Autodesk Fusion 360 part; units mm, degrees
sketch "Sketch6" plane through (0, 0, 0) normal (0, 1, 0) x (1, 0, 0)
  line L0 (0, 0) -> (-31.75, 0)
  line L1 (-31.75, 0) -> (-31.75, -7.62)
  line L2 (-31.75, -7.62) -> (0, -7.62)
  line L3 (0, -7.62) -> (0, 0)
  dimension "d16" = 7.62
  dimension "d17" = 31.75
extrude "Extrude5" add sketch "Sketch6" along normal blind 3
sketch "Sketch7" plane through (0, 0, 0) normal (0, -1, 0) x (1, 0, 0)
  line L0 (0, 0) -> (0, 7.62)
  line L1 (0, 7.62) -> (-31.75, 7.62)
  line L2 (-31.75, 7.62) -> (-31.75, 0)
  line L3 (-31.75, 0) -> (0, 0)
  circle A0 centre (-29.21, 4) radius 1.5
  circle A1 centre (-2.54, 3.81) radius 1.5
  line L4 (-31.75, 7.62) -> (-26.75, 7.62)
  line L5 (-26.75, 7.62) -> (-26.75, 0)
  line L6 (-26.75, 0) -> (-31.75, 0)
  line L7 (-31.75, 0) -> (-31.75, 7.62)
  line L8 (0, 0) -> (-5, 0)
  line L9 (-5, 0) -> (-5, 7.62)
  line L10 (-5, 7.62) -> (0, 7.62)
  line L11 (0, 7.62) -> (0, 0)
  line L12 (-31.75, 7.62) -> (-21.75, 7.62)
  line L13 (-21.75, 7.62) -> (-21.75, 0)
  line L14 (-21.75, 0) -> (-31.75, 0)
  line L15 (-31.75, 0) -> (-31.75, 7.62)
  line L16 (0, 0) -> (-10, 0)
  line L17 (-10, 0) -> (-10, 7.62)
  line L18 (-10, 7.62) -> (0, 7.62)
  line L19 (0, 7.62) -> (0, 0)
  dimension "d20" = 3
  dimension "d21" = 3
  dimension "d22" = 26.67
  dimension "d24" = 2.54
  dimension "d25" = 3.81
  dimension "d30" = 5
  dimension "d31" = 5
  dimension "d36" = 10
  dimension "d37" = 10
extrude "Extrude8" cut sketch "Sketch7" against normal blind 1 contours L1 L2 L3 L4 L5 L6 L7 L12 L14 L15
extrude "Extrude7" cut sketch "Sketch7" against normal blind 3 contours A1
extrude "Extrude6" cut sketch "Sketch7" against normal blind 3 contours A0
extrude "Extrude9" cut sketch "Sketch7" against normal blind 1 contours L0 L1 L3 L8 L9 L10 L11 L16 L18 L19
sketch "Sketch8" plane through (0, 3, 0) normal (0, 1, 0) x (-1, 0, 0)
  circle A0 centre (29.21, 4) radius 1.5
  circle A1 centre (2.54, 3.81) radius 1.5
  line L0 (0, 7.62) -> (0, 0)
  line L1 (0, 0) -> (31.75, 0)
  line L2 (31.75, 0) -> (31.75, 7.62)
  line L3 (31.75, 7.62) -> (0, 7.62)
sketch "Sketch9" plane through (0, 0, 7.62) normal (0, 0, 1) x (-1, 0, 0)
  line L0 (5, -1) -> (0, -1)
  line L1 (0, -1) -> (0, -3)
  line L2 (0, -3) -> (31.75, -3)
  line L3 (31.75, -3) -> (31.75, -1)
  line L4 (31.75, -1) -> (26.75, -1)
  line L5 (26.75, -1) -> (26.75, 0)
  line L6 (26.75, 0) -> (5, 0)
  line L7 (5, 0) -> (5, -1)
  line L8 (31.75, -3) -> (21.75, -3)
  line L9 (21.75, -3) -> (21.75, -2)
  line L10 (21.75, -2) -> (31.75, -2)
  line L11 (31.75, -2) -> (31.75, -3)
  line L12 (0, -3) -> (10, -3)
  line L13 (10, -3) -> (10, -2)
  line L14 (10, -2) -> (0, -2)
  line L15 (0, -2) -> (0, -3)
  line L16 (21.75, -3) -> (10, -3)
  line L17 (10, -3) -> (10, -2)
  line L18 (10, -2) -> (21.75, -2)
  line L19 (21.75, -2) -> (21.75, -3)
  line L20 (21.75, 0) -> (10, 0)
  line L21 (10, 0) -> (10, -1)
  line L22 (10, -1) -> (21.75, -1)
  line L23 (21.75, -1) -> (21.75, 0)
  dimension "d39" = 10
  dimension "d40" = 1
  dimension "d45" = 11.75
extrude "Extrude12" add sketch "Sketch9" along normal blind 9 contours L6 L20 L21 L22 L23
extrude "Extrude11" cut sketch "Sketch9" against normal blind 10 contours L1 L2 L12 L13 L14 L15 L17
extrude "Extrude10" cut sketch "Sketch9" against normal blind 10 contours L2 L3 L8 L9 L10 L11 L19
The listing builds one solid part. Answer for the finished solid, in the listing's coordinates (mm). A direction names the side the tool comes from. Coordinates: 2 decimals unless noted, no trailing zeros. Order: outer loops, then holes, each group sorted by start corner. A loop starts at its lowest first (then second) coordinate and runs counter-clockwise, first axis right, second up. Notation, with made-up numbers: (64.25, 14) -> (96.25, 14) arc R20 ccw to (96.25, 40) -> close; hole circle Ø7 at (-9.75, -25.5). An arc over 180 degrees is marked (long way). Answer in a Markdown table with one row per item. Add a question column.
Item 1: Each of these flat-tipped pins is pushed along its axis until it touches: P1, Ø2.5, axis at x = -30.5, z = 3.5, coming from the -Y side; P2, Ø1.5, axis at x = -15.5, z = 12, coming from the +Y side; P3, Ø4, axis at x = -2.54, z = 3.81, coming from the +Y side. Where does it stop, or does it pass through?
Item 2: Find section A-A (y = 0.4). Write down the section's boundary in (x, z), then the cut area to 3 significant figures.
Item 3: Find section B-B (x = -29.21). Write down the section's boundary in (y, z).
Item 4: Which of the six approach directions +Z, -Z, +X, -X, +Y, -Y give full straight-line access (tool end or side, diameter ignored) to faces 1 (the face through (-26.75, 0.5, 3.9)), 2 (the face through (-27, 2, 4)), 3 (the face through (-21.75, 0.5, 12.1)), 4 (the face through (-16, 1, 12)), 5 (the face through (-4.2, 1, 3.9))?
Item 5: Determine the mould class of faces 6 (the face through (0, 1.5, 3.9)), 7 (the face through (-2.7, 1.5, 5.3)), 8 (the face through (-5, 2, 4)), 9 (the face through (-31.75, 1.5, 3.8)) for opening direction X: +X half, -X half, draft (parallel to the pull), parting line (faces both ways), or undercut.
Item 6: Find section D-D (x = -15). Write down the section's boundary in (y, z).
Item 7: Find the intervals of material crossed by L1, parallel to Z at x = -29.21, y = 1.45; L2, parallel to Z at x = -2.54, y = 1.2; L3, parallel to Z at x = -10, y = 1.55, in increasing order. Write a range as from..to.
Item 8: Find section C-C (z = 1.5). Write down the section's boundary in (x, y).
Result set:
| question | item | result |
|---|---|---|
| 1 | P1 | stops at y = 1 |
| 1 | P2 | stops at y = 1 |
| 1 | P3 | stops at y = 2 |
| 2 | outline | (-26.75, 0) -> (-5, 0) -> (-5, 7.62) -> (-10, 7.62) -> (-10, 16.62) -> (-21.75, 16.62) -> (-21.75, 7.62) -> (-26.75, 7.62) -> close |
| 2 | area | 271 mm² |
| 3 | outline | (1, 0) -> (2, 0) -> (2, 2.5) -> (1, 2.5) -> close; (1, 5.5) -> (2, 5.5) -> (2, 7.62) -> (1, 7.62) -> close |
| 4 | face 1 | +Z, -Z, -X, -Y |
| 4 | face 2 | +Z, -Z, -X, +Y |
| 4 | face 3 | +Z, -X, +Y, -Y |
| 4 | face 4 | +Z, +X, -X, +Y |
| 4 | face 5 | +Z, -Z, +X, -Y |
| 5 | face 6 | +X half |
| 5 | face 7 | undercut |
| 5 | face 8 | draft |
| 5 | face 9 | -X half |
| 6 | outline | (0, 0) -> (3, 0) -> (3, 7.62) -> (1, 7.62) -> (1, 16.62) -> (0, 16.62) -> close |
| 7 | L1 | z = 0..2.5, 5.5..7.62 |
| 7 | L2 | z = 0..2.31, 5.31..7.62 |
| 7 | L3 | z = 0..7.62 |
| 8 | outline | (-31.75, 1) -> (-26.75, 1) -> (-26.75, 0) -> (-5, 0) -> (-5, 1) -> (0, 1) -> (0, 2) -> (-10, 2) -> (-10, 3) -> (-21.75, 3) -> (-21.75, 2) -> (-31.75, 2) -> close |
